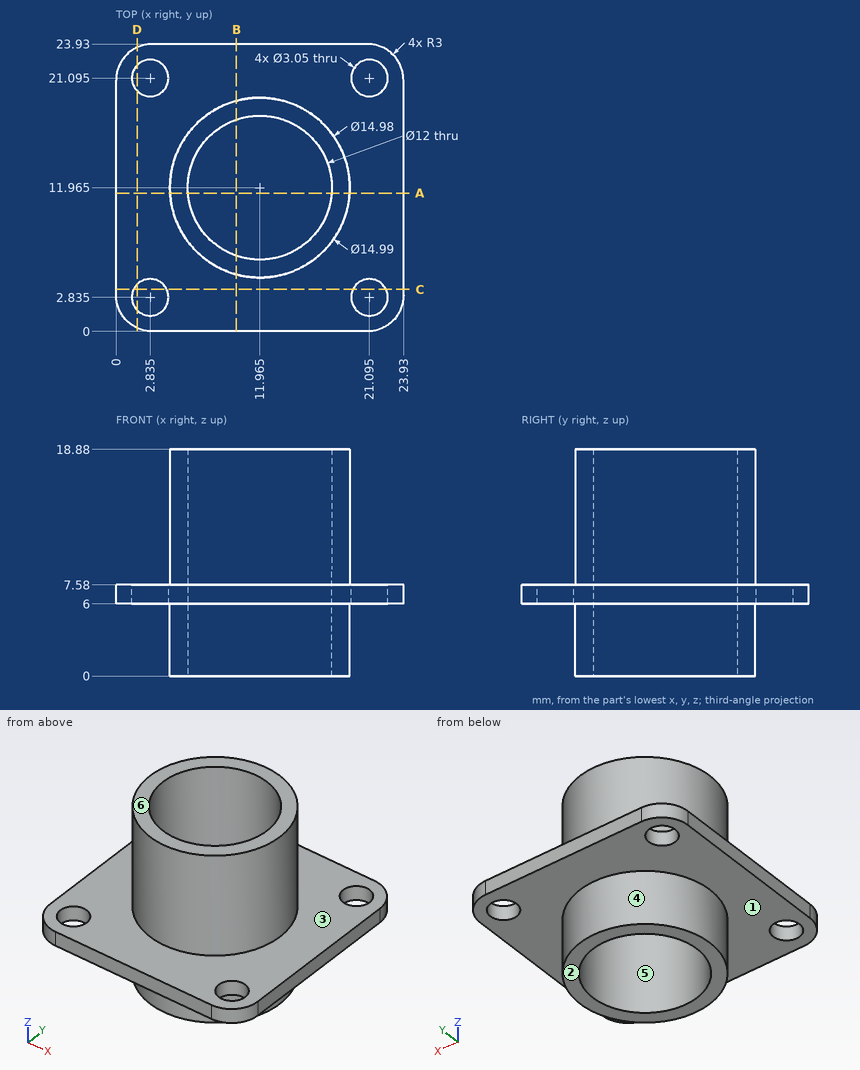
Study the drawing (mm; zero at the part's minimum x, y, z) and answer. A direction names the side the tool comes from. Coordinates: 2 decimals unless noted, no trailing zeros. Write each loop counter-clockwise with the first axis right and the second up, starting at its lowest first coordinate (ties: lowest second). Pieces come first, ordered by that corner, then holes. Notation, with made-up numbers: (57, 77) - (83, 77) arc R16 ccw to (83, 106) - close; hole circle Ø4 at (21.5, 2.25). An arc over 180 degrees is marked (long way). Return JSON: item names as keys, results as strings. Group by question number.
1. A cutting plane is placed at A-A, the plane y = 11.5. Determine the outline of the cut face in (x, z), plus the area to 3 significant figures.
2. A cutting plane is placed at B-B, the plane x = 10. Determine the outline of the cut face in (y, z).
3. Which of the six approach directions +Z, -Z, +X, -X, +Y, -Y give full straight-line access (tool end or side, diameter ignored) to the marked faces 1, 2 and 3?
4. A cutting plane is placed at D-D, the plane x = 1.75. Determine the outline of the cut face in (y, z).
5. Given pin 1 (4 mm diameter, centred on x = 21.095, y = 21.095, fed in from -Z); pin 2 (2 mm diameter, centred on x = 5, y = 19.5, fed in from +Z); pin 3 (10 mm diameter, centred on x = 18.5, z = 16, fed in from -Y), each flat-ended and moving along its own axis, determine where each tip first touches the part or whether it passes through.
6. Straight lines are drawn through the part: L1, parallel to Y at x = 12, z = 14.25; L2, parallel to Z at x = 4, y = 1.75. For each, find the intervals that lie inside material, in ascending order.
7. Determine the mould class of the marked faces 4, 5 and 6 for opening direction X: released by +X, released by -X, zero draft, split by the parting line, or undercut.
8. A cutting plane is placed at C-C, the plane y = 3.5. Determine the outline of the cut face in (x, z), plus the area to 3 significant figures.
Ans:
{
 "1": {"outline": "(0, 6) - (4.49, 6) - (4.49, 0) - (5.98, 0) - (5.98, 18.88) - (4.48, 18.88) - (4.48, 7.58) - (0, 7.58) - close; (17.95, 0) - (19.44, 0) - (19.44, 6) - (23.93, 6) - (23.93, 7.58) - (19.45, 7.58) - (19.45, 18.88) - (17.95, 18.88) - close", "area": "70.7 mm²"},
 "2": {"outline": "(0, 6) - (4.74, 6) - (4.74, 0) - (6.3, 0) - (6.3, 18.88) - (4.73, 18.88) - (4.73, 7.58) - (0, 7.58) - close; (17.63, 0) - (19.19, 0) - (19.19, 6) - (23.93, 6) - (23.93, 7.58) - (19.2, 7.58) - (19.2, 18.88) - (17.63, 18.88) - close"},
 "3": {"face 1": "-Z", "face 2": "-Z, +X, -X, +Y, -Y", "face 3": "+Z"},
 "4": {"outline": "(0.27, 6) - (1.76, 6) - (1.76, 7.58) - (0.27, 7.58) - close; (3.91, 6) - (20.02, 6) - (20.02, 7.58) - (3.91, 7.58) - close; (22.17, 6) - (23.66, 6) - (23.66, 7.58) - (22.17, 7.58) - close"},
 "5": {"pin 1": "z = 6", "pin 2": "z = 7.58", "pin 3": "y = 4.63"},
 "6": {"L1": "4.47 to 5.97, 17.96 to 19.46", "L2": "6 to 7.58"},
 "7": {"face 4": "split by the parting line", "face 5": "undercut", "face 6": "zero draft"},
 "8": {"outline": "(0, 6) - (1.46, 6) - (1.46, 7.58) - (0, 7.58) - close; (4.21, 6) - (19.72, 6) - (19.72, 7.58) - (4.21, 7.58) - close; (22.47, 6) - (23.93, 6) - (23.93, 7.58) - (22.47, 7.58) - close", "area": "29.1 mm²"}
}
